Could you check a few things on this model? Use its own coordinates, in mm. Coordinates: 2 decimals unless noted, no trailing zeros. Order: outer loops, then holes, each group sorted by start corner. A loop starts at its lowest first (then second) coordinate and runs counter-clockwise, first axis right, second up.
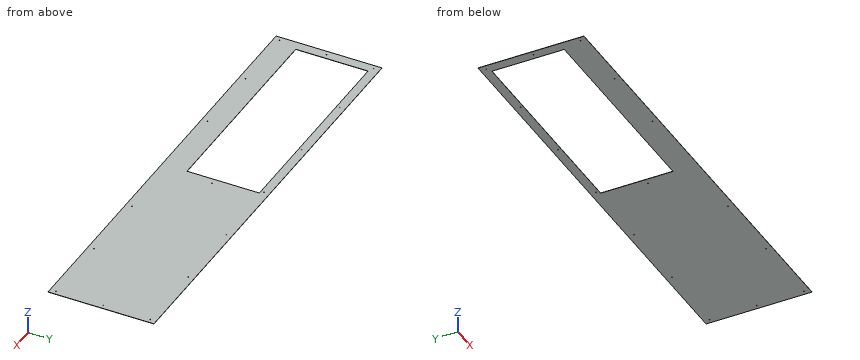
```python
from build123d import *

# Parameters (mm, degrees)
F0_W     = 1912.3025
F0_H     = 460.248
F0_W_2   = 911.5298
F0_H_2   = 314.325
F1_DEPTH = 0.9525
F2_R     = 1.905
F3_DEPTH = 25.4


with BuildPart() as f1:
    # F0 (on Top) → F1 (new body)
    with BuildSketch(Plane.XY):
        with Locations((-2.511288, -258.409424)):
            Rectangle(F0_W, F0_H)
        with Locations((-459.781138, -223.547924)):
            Rectangle(F0_W_2, F0_H_2, mode=Mode.SUBTRACT)
    extrude(amount=F1_DEPTH)

    # F2 (on face) → F3 (cut)
    with BuildSketch(Plane(origin=(0, 0, 0), x_dir=(1, 0, 0), z_dir=(0, 0, -1))):
        with Locations((934.589962, 53.685424)):
            Circle(F2_R)
        with Locations((617.089962, 53.685424)):
            Circle(F2_R)
        with Locations((299.589962, 53.685424)):
            Circle(F2_R)
        with Locations((-17.910038, 53.685424)):
            Circle(F2_R)
        with Locations((-335.410038, 53.685424)):
            Circle(F2_R)
        with Locations((-652.910038, 53.685424)):
            Circle(F2_R)
        with Locations((-938.672738, 53.685424)):
            Circle(F2_R)
        with Locations((934.589962, 258.345924)):
            Circle(F2_R)
        with Locations((934.589962, 463.133424)):
            Circle(F2_R)
        with Locations((-938.672738, 258.345924)):
            Circle(F2_R)
        with Locations((-938.672738, 463.133424)):
            Circle(F2_R)
        with Locations((-652.910038, 463.133424)):
            Circle(F2_R)
        with Locations((-335.410038, 463.133424)):
            Circle(F2_R)
        with Locations((299.589962, 463.133424)):
            Circle(F2_R)
        with Locations((617.089962, 463.133424)):
            Circle(F2_R)
        with Locations((21.510762, 258.345924)):
            Circle(F2_R)
    extrude(amount=-F3_DEPTH, mode=Mode.SUBTRACT)


solid = f1.part
```
Item 1: For pin 1 Ø5 at (x, y) = (934.59, -463.13) entering from -Z, with a flat end and sliding along its axis, tell me the tip position at first contact or that it passes through.
Item 2: I need wall thicknesses on line 1 (Y direction, x = -280.5, z = 0.7); line 2 (X direction, y = -292, z = 0.35). Which ranges of each line are inside material? Lowest first, please.
Item 3: Suppose I cut it at B-B (x = -128.5). List the corners of the cut face in (y, z) for me, and give its area (3 significant figures).
Item 4: Suppose I cut it at C-C (z = 0.15). Count the separate pieces of the cut face and the enclosed holes in it, and give its area (3 significant figures).
Item 5: Suppose I cut it at A-A (y = -99). List the corners of the cut face in (x, z) for me, and give its area (3 significant figures).
Geometry results:
1. pin 1: stops at z = 0
2. line 1: y = -488.53 to -380.71, -66.39 to -28.29
2. line 2: x = -958.66 to -915.55, -4.02 to 953.64
3. outline: (-488.53, 0) - (-380.71, 0) - (-380.71, 0.95) - (-488.53, 0.95) - close; (-66.39, 0) - (-28.29, 0) - (-28.29, 0.95) - (-66.39, 0.95) - close
3. area: 139 mm2
4. separate pieces: 1
4. enclosed holes: 17
4. area: 593,000 mm2
5. outline: (-958.66, 0) - (-915.55, 0) - (-915.55, 0.95) - (-958.66, 0.95) - close; (-4.02, 0) - (953.64, 0) - (953.64, 0.95) - (-4.02, 0.95) - close
5. area: 953 mm2
